CAD build for the part. Positions are in the model's coordinates, mm. A direction names the side the tool comes from. Round coordinates to 2 decimals unless told otherwise and drop trailing zeros. Loops run counter-clockwise (first coordinate to the right, second up) from the corner with the lowest first, then second, coordinate; pieces in that order, holes last. Notation, with made-up numbers: M 31,21.25 L 50,21.25 A16 ccw 50,46.25 Z; hole C 4,-15 d3. An arc over 180 degrees is marked long. Put each result on its own line as item: value. Start each with the question number.
from build123d import *

# Parameters (mm, degrees)
SKETCH_1_W      = 5
SKETCH_1_H      = 2
EXTRUDE_1_DEPTH = 4
EXTRUDE_2_DEPTH = 1
EXTRUDE_3_DEPTH = 2


with BuildPart() as part:
    # Sketch 1 → Extrude 1 (new body)
    with BuildSketch(Plane(origin=(0, 0, 0), x_dir=(1, 0, 0), z_dir=(0, 1, 0))):
        with Locations((2.5, 1)):
            Rectangle(SKETCH_1_W, SKETCH_1_H)
    extrude(amount=EXTRUDE_1_DEPTH)

    # Sketch 1_3 → Extrude 2 (add)
    with BuildSketch(Plane(origin=(0, 0, 0), x_dir=(1, 0, 0), z_dir=(0, 1, 0))):
        Polygon((6, -2), (6, 0), (5, 0), (0, 0), (0, -2), align=None)
    extrude(amount=EXTRUDE_2_DEPTH)

    # Sketch 2 → Extrude 3 (add)
    with BuildSketch(Plane(origin=(6, 0, 0), x_dir=(0, 0, -1), z_dir=(1, 0, 0))):
        Polygon((-1, 1), (0, 1), (0, 3), (-2, 3), (-2, 2), (-1, 2), align=None)
    extrude(amount=-EXTRUDE_3_DEPTH)


solid = part.part
(1) Cut at B-B on x = 5.65. List the corners of the cut face in (y, z), and give its area (3 significant figures).
(2) Mould opens along Y. For faces 1 (the flat face through (4, 2.2, 0.8)), 2 (the flat face through (5, 3, 1)), 3 (the flat face through (5, 2, 1.5)), 4 (the flat face through (2, 1, 1)) say: +Y half, -Y half, draft (parallel to the pull), parting line (faces both ways), or undercut.
(3) Tool access for faces 5 (the flat face through (5.5, 1.5, 0)), 6 (the flat face through (5, 1.5, 1)), 7 (the flat face through (3, 0, 0)): list every direction of +Z, -Z, +X, -X, +Y, -Y with a clear straight run to the whole face (end or side of a thin tool).
(4) Cut at D-D on z = 0.3. List the corners of the cut face in (x, y), and give its area (3 significant figures).
(5) Flat gauge pins, fed straight in: pin 1 Ø1.1 at (x, z) = (5.5, 1.5) entering from -Y; pin 2 Ø0.6 at (x, z) = (5, 1.5) entering from +Y; pin 3 Ø1 at (x, z) = (2, 1.5) entering from +Y; pin 4 Ø0.6 at (y, z) = (1.5, -1) entering from +X. Where does each tip first touch, or does it go through?
(6) Drill centre lines: line 1 along Z through (x, y) = (1.65, 1.4); line 2 along X through (y, z) = (2.95, 0.9); line 3 along X through (y, z) = (2.1, -1.65). Where is each one in solid material? Low to high.
(7) Cut at A-A on z = 1.2. List the corners of the cut face in (x, y).
(8) Cut at C-C on y = 1.6. List the corners of the cut face in (x, z).
Taken from the geometry:
1. outline: M 0,0 L 3,0 L 3,2 L 2,2 L 2,1 L 1,1 L 1,2 L 0,2 Z
1. area: 5.00 mm2
2. face 1: draft
2. face 2: +Y half
2. face 3: undercut
2. face 4: undercut
3. face 5: -Z, +X, +Y, -Y
3. face 6: +Z, +X, -X
3. face 7: +Z, -Z, +X, -X, -Y
4. outline: M 0,0 L 6,0 L 6,3 L 4,3 L 4,1 L 0,1 Z
4. area: 10.0 mm2
5. pin 1: y = 0
5. pin 2: y = 3
5. pin 3: y = 1
5. pin 4: x = 5
6. line 1: -2 to 0
6. line 2: 4 to 6
6. line 3: 0 to 5
7. outline: M 0,0 L 6,0 L 6,1 L 0,1 Z; M 4,2 L 6,2 L 6,3 L 4,3 Z
8. outline: M 0,-2 L 5,-2 L 5,0 L 6,0 L 6,1 L 4,1 L 4,0 L 0,0 Z
